Input: dimensioned drawing with shaded views. Units: mm. Origin: part minimum x, y, z. A direction names the side the tool comes from. Give positions to 0.01 mm unless a question says otherwise; leave off trailing zeros. Write each loop counter-clockwise with the first axis right and the second up, starting at its lowest first coordinate (ties: lowest second). Pieces come first, ordered by that corner, then holes.
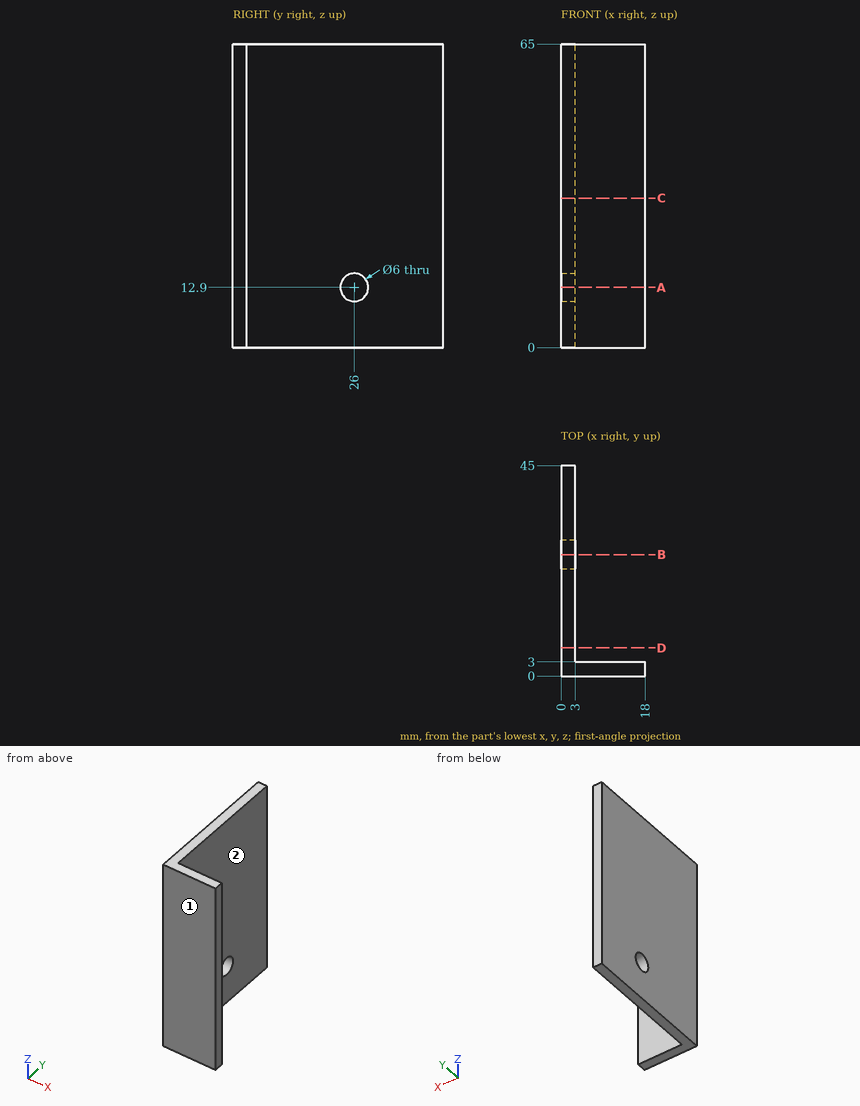
Item 1: Section B-B, the plane y = 26. Return the cut outline in (x, z), plus the area to 3 significant figures.
Found:
outline: (0, 0) - (3, 0) - (3, 9.9) - (0, 9.9) - close; (0, 15.9) - (3, 15.9) - (3, 65) - (0, 65) - close
area: 177 mm2
Item 2: Pin query (flat end, axial travel): pin 1 Ø2 at (y, z) = (14.5, 58.5) entering from +X; pin 2 Ø5 at (y, z) = (13.5, 44.5) entering from -X; pin 3 Ø7.5 at (x, z) = (10.5, 24.5) entering from +Y; pin 4 Ø3.5 at (y, z) = (26, 12.9) entering from -X. Return the tip coordinate at first contact, or that it passes through.
Found:
pin 1: stops at x = 3
pin 2: stops at x = 0
pin 3: stops at y = 3
pin 4: passes through
Item 3: Section C-C, the plane z = 32. Return the cut outline in (x, y).
Found:
outline: (0, 0) - (18, 0) - (18, 3) - (3, 3) - (3, 45) - (0, 45) - close
Item 4: Section D-D, the plane y = 6. Return the cut outline in (x, z), plus the area to 3 significant figures.
Found:
outline: (0, 0) - (3, 0) - (3, 65) - (0, 65) - close
area: 195 mm2
Item 5: Line query: L1, parallel to Z at x = 0.75, y = 26; L2, parallel to X at y = 7.5, z = 17. Output: solid intervals per line, ascending.
Found:
L1: z = 0 to 9.9, 15.9 to 65
L2: x = 0 to 3
Item 6: Reachability of the marked faces 1 and 2 from +Z, -Z, +X, -X, +Y, -Y: full face, straight path, thin tool, end or side. Return the list, or none.
Found:
face 1: +Z, -Z, +X, -X, -Y
face 2: +Z, -Z, +X, +Y
Item 7: Section A-A, the plane z = 12.9. Return the cut outline in (x, y), plus the area to 3 significant figures.
Found:
outline: (0, 0) - (18, 0) - (18, 3) - (3, 3) - (3, 23) - (0, 23) - close; (0, 29) - (3, 29) - (3, 45) - (0, 45) - close
area: 162 mm2
